Model file for the job. Use its own axes, mm. A direction names the side the tool comes from. Round coordinates to 2 decimals unless told otherwise and drop trailing zeros. Loops run counter-clockwise (first coordinate to the right, second up) from the corner with the lowest first, then second, coordinate; pieces in that order, holes last.
from build123d import *

# Parameters (mm, degrees)
SKETCH2_R                         = 7.14375
CUT_EXTRUDE1_DEPTH                = 120.65
SKETCH5_W                         = 17
SKETCH5_H                         = 17
BOSS_EXTRUDE3_DEPTH               = 5
SKETCH4_R                         = 3
CUT_EXTRUDE2_DEPTH                = 139.35
FILLET1_R                         = 1
FILLET2_R                         = 0.25
F_1_4_20_TAPPED_HOLE1_D           = 5.1054
F_1_4_20_TAPPED_HOLE1_CSINK_D     = 7.62
F_1_4_20_TAPPED_HOLE1_CSINK_ANGLE = 100


with BuildPart() as part:
    # Sketch1 → Revolve1 (revolve)
    with BuildSketch(Plane.XY):
        Polygon((0, 0), (38.1, 0), (38.1, 6.35), (7.9375, 6.35), (7.9375, 133.35), (0, 133.35), align=None)
    revolve(axis=Axis((0, 131.17698584, 0), (0, -1, 0)))

    # Sketch2 → Cut-Extrude1 (cut)
    with BuildSketch(Plane(origin=(0, 0, 0), x_dir=(1, 0, 0), z_dir=(0, 1, 0))):
        Circle(SKETCH2_R)
    extrude(amount=CUT_EXTRUDE1_DEPTH, mode=Mode.SUBTRACT)

    # Sketch5 → Boss-Extrude3 (add)
    with BuildSketch(Plane(origin=(0, 133.35, 0), x_dir=(1, 0, 0), z_dir=(0, 1, 0))):
        Rectangle(SKETCH5_W, SKETCH5_H)
    extrude(amount=BOSS_EXTRUDE3_DEPTH)

    # Sketch4 → Cut-Extrude2 (cut, through all)
    with BuildSketch(Plane(origin=(0, 138.35, 0), x_dir=(1, 0, 0), z_dir=(0, 1, 0))):
        Circle(SKETCH4_R)
    extrude(amount=-CUT_EXTRUDE2_DEPTH, mode=Mode.SUBTRACT)

    # Fillet1
    fillet1_edges = [part.edges().sort_by_distance(p)[0] for p in [
        (8.5, 135.85, 8.5),
        (8.5, 135.85, -8.5),
        (-8.5, 135.85, -8.5),
        (-8.5, 135.85, 8.5),
    ]]
    fillet(fillet1_edges, radius=FILLET1_R)

    # Fillet2
    fillet2_edges = [part.edges().sort_by_distance(p)[0] for p in [
        (-7.9375, 133.35, 0),
    ]]
    fillet(fillet2_edges, radius=FILLET2_R)

    # 1/4-20 Tapped Hole1 (through all)
    with Locations(Plane(origin=(0, 6.35, 0), x_dir=(1, 0, 0), z_dir=(0, 1, 0))):
        with Locations((-13.139703049, -21.737253823), (-12.255162495, 22.24794355), (25.394865544, -0.510689727)):
            CounterSinkHole(F_1_4_20_TAPPED_HOLE1_D / 2, F_1_4_20_TAPPED_HOLE1_CSINK_D / 2, counter_sink_angle=F_1_4_20_TAPPED_HOLE1_CSINK_ANGLE)


solid = part.part
Q1. Slice it at C-C on z = 29.5. Give the cut face in (x, y).
Q2. Slice it at A-A on x = 0. Give the cut face in (y, z).
Q3. Slice it at D-D on x = -29.5. Give the cut face in (y, z).
Q4. Flat gauge pins, fed straight in: P1, Ø12, axis at y = 114.5, z = 11, coming from the +X side; P2, Ø1.5, axis at x = -2, y = 136, coming from the -Z side; P3, Ø4.5, axis at x = -12.26, z = -22.25, coming from the -Y side; P4, Ø1.5, axis at x = 0, y = 135.5, coming from the +Z side. Where does each tip first touch, or does it go through?
Q5. Probe line 1 (Y direction, x = 8, z = -2.5); line 2 (Z direction, x = 0, y = 132.75); line 3 (Y direction, x = 35, z = 14.5). List the from-to ranges inside material, lowest first.
Q6. Tool access for faces 1 (the face through (8.5, 136, 0)), 2 (the face through (-8, 133.35, -3)), 3 (the face through (-7.137, 59.48, -0.314)), 4 (the face through (0, 136, -8.5)), 5 (the face through (-8.5, 136, 0)): list every direction of +Z, -Z, +X, -X, +Y, -Y with a clear straight run to the whole face (end or side of a thin tool).
Q7. Slice it at B-B on y = 104.5. Give the cut face in (x, z) (1 decimal).
Q8. Pull direction X, two halves, no side cores. Call faces 6 (the face through (-1.72, 70.61, -7.75)), 7 (the face through (3, 120.65, 1)), 8 (the face through (-9, 6.35, 1)): pulls with the +X half, pulls with the -X half, needs draft (parallel to the pull), parting line crosses it, or undercut.
Reply:
1. outline: (-24.11, 0) - (24.11, 0) - (24.11, 6.35) - (-24.11, 6.35) - close
2. outline: (0, -38.1) - (6.35, -38.1) - (6.35, -7.94) - (133.1, -7.94) arc R0.25 cw to (133.35, -8.19) - (133.35, -8.5) - (138.35, -8.5) - (138.35, -3) - (120.65, -3) - (120.65, -7.14) - (0, -7.14) - close; (0, 7.14) - (120.65, 7.14) - (120.65, 3) - (138.35, 3) - (138.35, 8.5) - (133.35, 8.5) - (133.35, 8.19) arc R0.25 cw to (133.1, 7.94) - (6.35, 7.94) - (6.35, 38.1) - (0, 38.1) - close
3. outline: (0, -24.11) - (6.35, -24.11) - (6.35, 24.11) - (0, 24.11) - close
4. P1: stops at x = 6.16
4. P2: stops at z = -8.5
4. P3: passes through
4. P4: stops at z = 8.5
5. line 1: y = 0 to 6.35, 133.35 to 138.35
5. line 2: z = -7.94 to -3, 3 to 7.94
5. line 3: y = 0 to 6.35
6. face 1: +Z, -Z, +X, +Y
6. face 2: none
6. face 3: -Y
6. face 4: -Z, +X, -X, +Y
6. face 5: +Z, -Z, -X, +Y
7. outline: circle Ø15.9 at (0, 0); hole circle Ø14.3 at (0, 0)
8. face 6: parting line crosses it
8. face 7: undercut
8. face 8: needs draft
